Job drawing, mm, ordinate dimensions from the low corner. One solid piece. A direction names the side the tool comes from. Round coordinates to 2 decimals unless told otherwise and drop trailing zeros. Order: outer loops, then holes, each group sorted by start corner. A loop starts at its lowest first (then second) coordinate and runs counter-clockwise, first axis right, second up. Notation, with made-up numbers: (15, 74.25) -> (34, 74.25) arc R19 ccw to (34, 95.25) -> close; hole circle Ø1 at (-38, 67). An arc over 180 degrees is marked (long way). Answer as a JSON object with one key per item and string values. Group by question number.
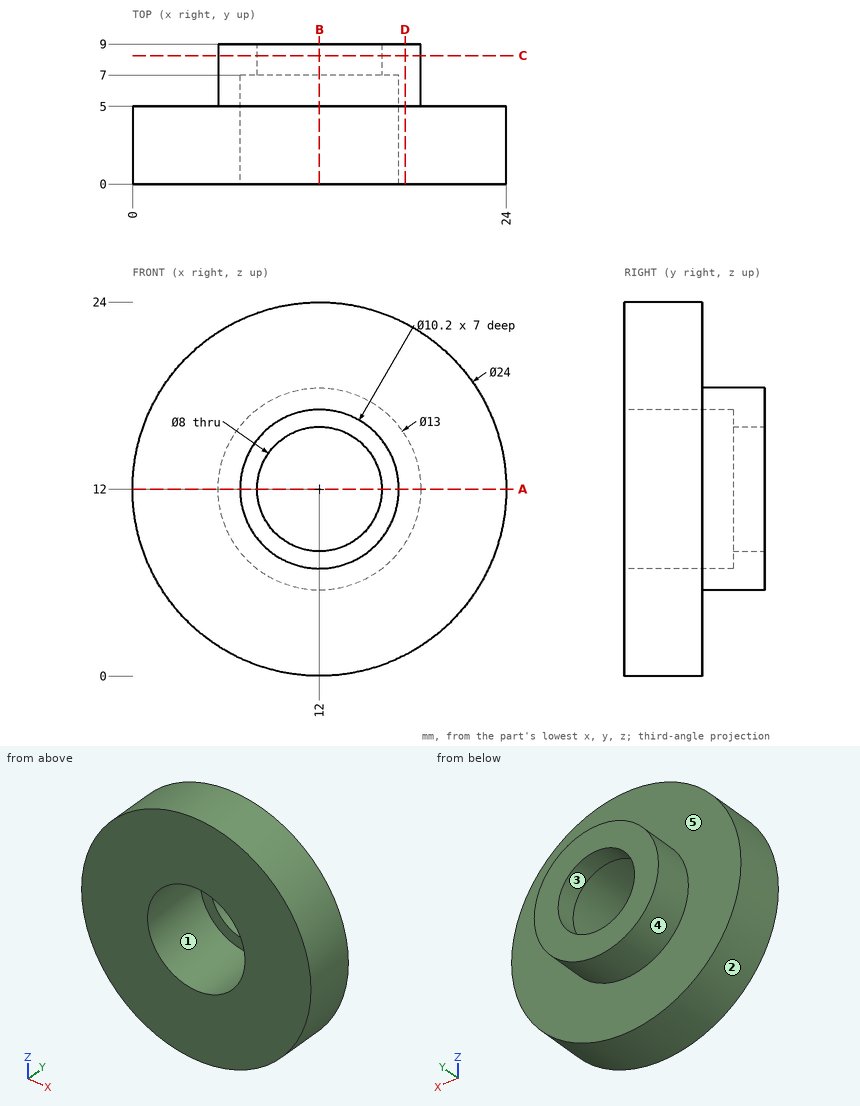
Q1. Two-plate mould, pull along Z, no slides. Class the marked faces 3, 4 and 5: +Z half, -Z half, draft (parallel to the pull), parting line (faces both ways), or undercut.
Q2. Band-saw the part on D-D (x = 17.5). List the corners of the cut face in (y, z).
Q3. Which spindle directions (+Z, -Z, +X, -X, +Y, -Y) get a long thin tool onto all of the face, cutting with end or side? Do the marked faces 1 and 2. Say none if no direction does.
Q4. Wall check: line 1 (X direction, y = 7.85, z = 12); line 2 (Z direction, x = 12, y = 2.25). Give the ranges that are in metal, low to high. Write a range as [from, to].
Q5. Drop flat-ended pins along their axis: pin 1 Ø2 at (y, z) = (7.5, 2.5) entering from -X; pin 2 Ø3 at (x, z) = (20.5, 13.5) entering from +Y; pin 3 Ø5 at (x, y) = (16.5, 5) entering from +Z; pin 4 Ø2 at (y, z) = (4, 18) entering from -X. Give the stop position or say it passes through.
Q6. Band-saw the part on B-B (x = 12). List the corners of the cut face in (y, z), plus the area to 3 significant figures.
Q7. Band-saw the part on A-A (z = 12). List the corners of the cut face in (x, y), plus the area to 3 significant figures.
Q8. Band-saw the part on C-C (y = 8.25). List the corners of the cut face in (x, z).
Completed:
{
 "1": {"face 3": "undercut", "face 4": "parting line", "face 5": "draft"},
 "2": {"outline": "(0, 1.33) -> (5, 1.33) -> (5, 8.54) -> (9, 8.54) -> (9, 15.46) -> (5, 15.46) -> (5, 22.67) -> (0, 22.67) -> close"},
 "3": {"face 1": "-Y", "face 2": "+Y, -Y"},
 "4": {"line 1": "[5.5, 8], [16, 18.5]", "line 2": "[0, 6.9], [17.1, 24]"},
 "5": {"pin 1": "through", "pin 2": "y = 5", "pin 3": "z = 23.83", "pin 4": "x = 1.09"},
 "6": {"outline": "(0, 0) -> (5, 0) -> (5, 5.5) -> (9, 5.5) -> (9, 8) -> (7, 8) -> (7, 6.9) -> (0, 6.9) -> close; (0, 17.1) -> (7, 17.1) -> (7, 16) -> (9, 16) -> (9, 18.5) -> (5, 18.5) -> (5, 24) -> (0, 24) -> close", "area": "84.6 mm2"},
 "7": {"outline": "(0, 0) -> (6.9, 0) -> (6.9, 7) -> (8, 7) -> (8, 9) -> (5.5, 9) -> (5.5, 5) -> (0, 5) -> close; (16, 7) -> (17.1, 7) -> (17.1, 0) -> (24, 0) -> (24, 5) -> (18.5, 5) -> (18.5, 9) -> (16, 9) -> close", "area": "84.6 mm2"},
 "8": {"outline": "circle Ø13 at (12, 12); hole circle Ø8 at (12, 12)"}
}
